from build123d import *

# Parameters (mm, degrees)
F0_W     = 69.85
F0_H     = 38.1
F1_DEPTH = 12.7
F2_W     = 12.7
F2_H     = 12.7
F3_DEPTH = 38.1
F5_DEPTH = 12.7
F6_R     = 6.35
F7_DEPTH = 12.7
F9_DEPTH = 12.7


with BuildPart() as f1:
    # F0 (on Top) → F1 (new body)
    with BuildSketch(Plane.XY):
        with Locations((68.010411, -20.100126)):
            Rectangle(F0_W, F0_H)
    extrude(amount=F1_DEPTH)

    # F2 (on face) → F3 (join)
    with BuildSketch(Plane.XZ.offset(39.150126)):
        with Locations((39.435411, -6.35)):
            Rectangle(F2_W, F2_H)
    extrude(amount=-F3_DEPTH)

    # F4 (on face) → F5 (cut)
    with BuildSketch(Plane.XY.offset(12.7)):
        with BuildLine():
            ThreePointArc((83.885411, -1.050126), (97.355795, -6.629742), (102.935411, -20.100126))
            Line((102.935411, -20.100126), (102.935411, -1.050126))
            Line((102.935411, -1.050126), (83.885411, -1.050126))
        make_face()
        with BuildLine():
            Line((102.935411, -39.150126), (102.935411, -20.100126))
            ThreePointArc((102.935411, -20.100126), (97.355795, -33.57051), (83.885411, -39.150126))
            Line((83.885411, -39.150126), (102.935411, -39.150126))
        make_face()
    extrude(amount=-F5_DEPTH, mode=Mode.SUBTRACT)

    # F6 (on face) → F7 (cut)
    with BuildSketch(Plane.XY.offset(12.7)):
        with Locations((83.885411, -20.100126)):
            Circle(F6_R)
    extrude(amount=-F7_DEPTH, mode=Mode.SUBTRACT)

    # F8 (on face) → F9 (join)
    with BuildSketch(Plane(origin=(0, -1.050126, 0), x_dir=(-1, 0, 0), z_dir=(0, 1, 0))):
        with BuildLine():
            ThreePointArc((-58.485411, 12.7), (-58.409892, 14.082925), (-58.184233, 15.449404))
            ThreePointArc((-58.184233, 15.449404), (-59.164143, 13.706609), (-60.891655, 12.7))
            Line((-60.891655, 12.7), (-58.485411, 12.7))
        make_face()
        with BuildLine():
            Line((-58.485411, 12.7), (-33.085411, 12.7))
            ThreePointArc((-33.085411, 12.7), (-44.402486, 25.324481), (-58.184233, 15.449404))
            ThreePointArc((-58.184233, 15.449404), (-58.409892, 14.082925), (-58.485411, 12.7))
        make_face()
    extrude(amount=-F9_DEPTH)


solid = f1.part
Geometry: final body of the model. Coordinates: model frame, mm. A direction names the side the tool comes from. Give positions to 0.01 mm unless a question says otherwise; leave off trailing zeros. Order: outer loops, then holes, each group sorted by start corner. A loop starts at its lowest first (then second) coordinate and runs counter-clockwise, first axis right, second up. Notation, with made-up numbers: (48, 77.5) -> (84, 77.5) arc R13 cw to (84, 92.5) -> close; hole circle Ø9 at (-19.5, 62.25). An arc over 180 degrees is marked (long way). Put each result on its own line as item: value.
Q1. Section C-C, the plane x = 66.5. Return loops of the section in (y, z).
Here are the results:
outline: (-39.15, 0) -> (-1.05, 0) -> (-1.05, 12.7) -> (-39.15, 12.7) -> close
Q2. Pin query (flat end, axial travel): pin 1 (6.5 mm diameter, centred on x = 46, z = 20.5, fed in from -Y); pin 2 (19 mm diameter, centred on x = 82.5, y = -28.5, fed in from +Z); pin 3 (4 mm diameter, centred on y = -20.5, z = -8.5, fed in from +X). Return the tip coordinate at first contact, or that it passes through.
Here are the results:
pin 1: stops at y = -13.75
pin 2: stops at z = 12.7
pin 3: stops at x = 45.79
Q3. Reachability of faces 1 (the face through (59.14, -7.31, 13.73)), 2 (the face through (47, -13.75, 18)), 3 (the face through (68, -24, 12.7)), 4 (the face through (74, -20, 0)) from +Z, -Z, +X, -X, +Y, -Y: full face, straight path, thin tool, end or side. Return the list, or none.
Here are the results:
face 1: +Z, +X, +Y, -Y
face 2: +Z, +X, -X, -Y
face 3: +Z, +X, -Y
face 4: -Z, +X, +Y, -Y
Q4. Section B-B, the plane y = -12. Return loops of the section in (x, z).
Here are the results:
outline: (33.09, -12.7) -> (45.79, -12.7) -> (45.79, 0) -> (101.13, 0) -> (101.13, 12.7) -> (60.89, 12.7) arc R3.81 cw to (58.18, 15.45) arc R12.7 ccw to (33.09, 12.7) -> close
Q5. Section D-D, the plane z = -2. Return loops of the section in (x, y), then the cut area to 3 significant figures.
Here are the results:
outline: (33.09, -39.15) -> (45.79, -39.15) -> (45.79, -1.05) -> (33.09, -1.05) -> close
area: 484 mm^2
Q6. Material intervals for L1, parallel to X at y = -28, z = -11; L2, parallel to Z at x = 98.5, y = -17.5; L3, parallel to Y at x = 37.5, z = 20, sorted ascending.
Here are the results:
L1: x = 33.09 to 45.79
L2: z = 0 to 12.7
L3: y = -13.75 to -1.05
Q7. Section A-A, the plane z = 3. Return loops of the section in (x, y).
Here are the results:
outline: (33.09, -39.15) -> (83.89, -39.15) arc R19.05 ccw to (102.94, -20.1) arc R19.05 ccw to (83.89, -1.05) -> (33.09, -1.05) -> close; hole circle Ø12.7 at (83.89, -20.1)
